Can you work these out from the model? Positions are in its coordinate system, mm. A direction names the side the tool comes from. Coordinates: 2 decimals unless noted, no trailing zeros. Order: outer loops, then holes, each group sorted by start corner. A loop starts at its lowest first (then second) coordinate and runs counter-clockwise, first axis right, second up. Notation, with made-up numbers: M 2,-22.75 L 35,-22.75 A13 cw 35,-11.75 Z; hole C 53,-27 d2. An arc over 180 degrees is marked long. Answer as a JSON object with one key per item and string values.
from build123d import *

# Parameters (mm, degrees)
SKETCH_1_R               = 60
SKETCH_1_R_2             = 10
EXTRUDE_1_DEPTH          = 10
CUT_EXTRUDE_1_DEPTH      = 121
PATTERN_CIRCULAR_1_COUNT = 4


with BuildPart() as part:
    # 草图1 → 凸台-拉伸1 (new body)
    with BuildSketch(Plane.XY):
        Circle(SKETCH_1_R)
        Circle(SKETCH_1_R_2, mode=Mode.SUBTRACT)
    extrude(amount=EXTRUDE_1_DEPTH)

    # 草图2 → 切除-拉伸1 (cut, symmetric)
    with BuildSketch(Plane.XY):
        with BuildLine():
            Line((0, 50), (0, 20))
            ThreePointArc((0, 20), (10, 17.320508076), (17.320508076, 10))
            Line((17.320508076, 10), (43.301270189, 25))
            ThreePointArc((43.301270189, 25), (25, 43.301270189), (0, 50))
        make_face()
    cut_extrude_1 = extrude(amount=CUT_EXTRUDE_1_DEPTH, both=True, mode=Mode.SUBTRACT)

    # 阵列(圆周)1: 切除-拉伸1 ×4 about axis
    pattern_circular_1_axis = Axis((0, 0, 10.5), (0, 0, -1))
    for i in range(1, PATTERN_CIRCULAR_1_COUNT):
        add(cut_extrude_1.rotate(pattern_circular_1_axis, i * 360 / PATTERN_CIRCULAR_1_COUNT), mode=Mode.SUBTRACT)


solid = part.part
Item 1: I want a section at B-B, the plane x = 27. Write out the boundary of the cut face in (y, z), plus the area to 3 significant figures.
Answers follow:
{"outline": "M -53.58,0 L -42.08,0 L -42.08,10 L -53.58,10 Z; M 0,0 L 15.59,0 L 15.59,10 L 0,10 Z; M 42.08,0 L 53.58,0 L 53.58,10 L 42.08,10 Z", "area": "386 mm^2"}
Item 2: Which directions (+Z, -Z, +X, -X, +Y, -Y) give clear straight access to the entire face, cutting with the end or side of a thin tool? Please do faces 1 (the flat face through (12, 1, 0)), 2 (the flat face through (17.395, -30.129, 5.07)).
Answers follow:
{"face 1": "-Z, +X, -X, +Y, -Y", "face 2": "+Z, -Z"}
Item 3: I want a section at A-A, the plane y = 41.5. Write out the boundary of the cut face in (x, z), plus the area to 3 significant figures.
Answers follow:
{"outline": "M -43.33,0 L -27.89,0 L -27.89,10 L -43.33,10 Z; M -23.96,0 L 0,0 L 0,10 L -23.96,10 Z; M 27.89,0 L 43.33,0 L 43.33,10 L 27.89,10 Z", "area": "548 mm^2"}
Item 4: If we mould it in two halves opening along X, with no side actions, what happens to faces 3 (the cylindrical face through (-59.94, 2.64, 4.93)), 4 (the flat face through (12, 1, 10)), 5 (the cylindrical face through (-25.317, -43.117, 5.07))? For each: pulls with the +X half, pulls with the -X half, needs draft (parallel to the pull), parting line crosses it, or undercut.
Answers follow:
{"face 3": "parting line crosses it", "face 4": "needs draft", "face 5": "undercut"}
Item 5: I want a section at D-D, the plane y = -45. Write out the boundary of the cut face in (x, z).
Answers follow:
{"outline": "M -39.69,0 L -21.79,0 L -21.79,10 L -39.69,10 Z; M 0,0 L 39.69,0 L 39.69,10 L 0,10 Z"}
Item 6: I'm going to push flat-ended pins straight in: pin 1 (8 mm diameter, centred on x = 29.5, y = 20, fed in from +Z); pin 2 (5 mm diameter, centred on y = -28.5, z = 6, fed in from -X); pin 3 (4 mm diameter, centred on y = 7, z = 2.5, fed in from -X); pin 4 (5 mm diameter, centred on x = 40, z = 2.5, fed in from -Y). Where does each tip first touch, or does it pass through?
Answers follow:
{"pin 1": "stops at z = 10", "pin 2": "stops at x = -54.07", "pin 3": "stops at x = -59.79", "pin 4": "stops at y = -46.84"}
Item 7: Please list where these lines run through material, in increasing order: line 1 (X direction, y = 22.5, z = 0.5); line 2 (Y direction, x = 14, z = 7); line 3 (X direction, y = 36.5, z = 9.25).
Answers follow:
{"line 1": "x = -55.62 to -44.65, -12.99 to 0, 38.97 to 55.62", "line 2": "y = -58.34 to -24.25, -14.28 to 14.28, 48 to 58.34", "line 3": "x = -47.62 to -34.17, -21.07 to 0, 34.17 to 47.62"}
Item 8: I want a section at C-C, the plane z = 3.5. Write out the boundary of the cut face in (x, y), plus the area to 3 significant figures.
Answers follow:
{"outline": "C 0,0 d120; hole M -50,0 L -20,0 A20 cw -10,17.32 L -25,43.3 A50 ccw Z; hole M -43.3,-25 A50 ccw 0,-50 L 0,-20 A20 cw -17.32,-10 Z; hole C 0,0 d20; hole M 0,20 A20 cw 17.32,10 L 43.3,25 A50 ccw 0,50 Z; hole M 10,-17.32 L 25,-43.3 A50 ccw 50,0 L 20,0 A20 cw Z", "area": "6,600 mm^2"}
